Geometry: see drawing. Coordinates: mm, zero at the bounding-box minimum. A direction names the side the tool comes from. Give positions to 0.01 mm unless a question says otherwise; leave off trailing zeros. Write each loop counter-clockwise with the first axis right and the second up, starting at its lowest first coordinate (ties: lowest second). Pieces come first, ordered by that corner, then holes. Notation, with made-up numbers: (49, 52) - (76, 52) arc R33 cw to (76, 85) - close; hole circle Ø3 at (58, 43.5). An arc over 180 degrees is marked (long way). Return JSON: item names as keys, results as strings.
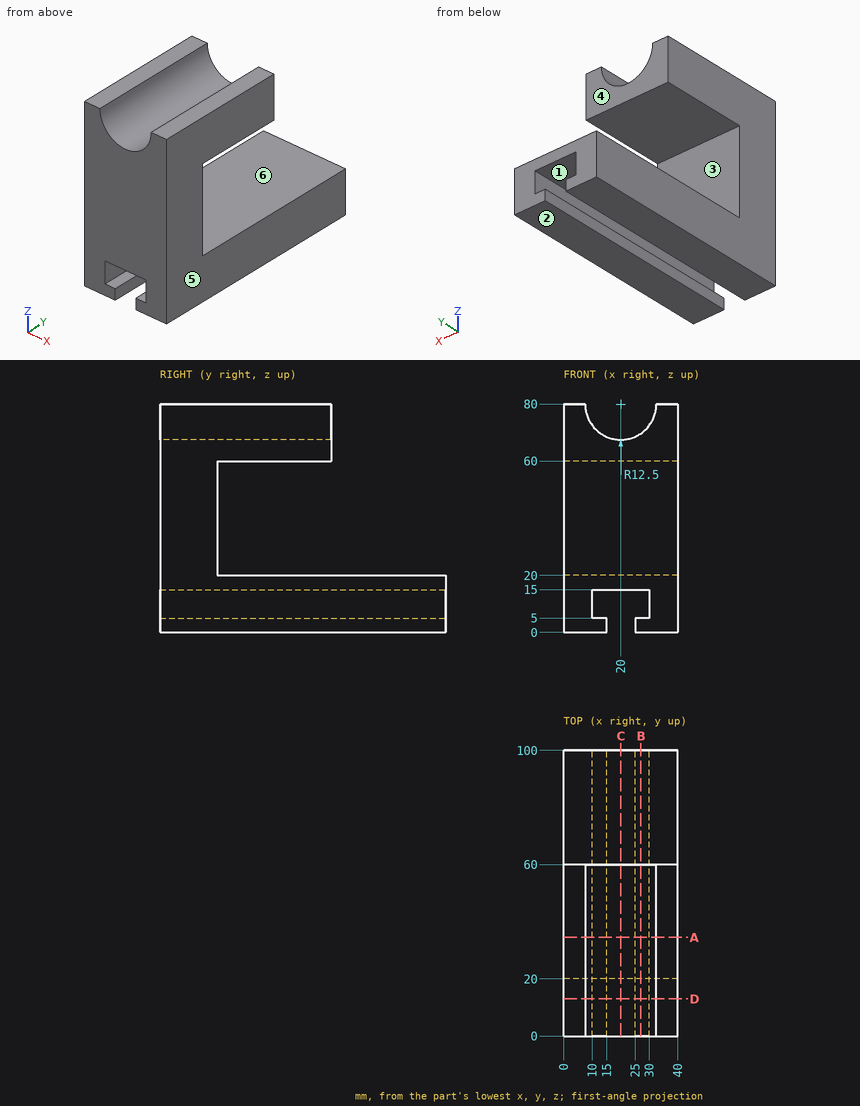
Q1. Section query D-D, the plane y = 13. Return the cut outline in (x, z).
Answer key:
{"outline": "(0, 0) - (15, 0) - (15, 5) - (10, 5) - (10, 15) - (30, 15) - (30, 5) - (25, 5) - (25, 0) - (40, 0) - (40, 80) - (32.5, 80) arc R12.5 cw to (7.5, 80) - (0, 80) - close"}
Q2. Section query B-B, the plane x = 27. Return the cut outline in (y, z).
Answer key:
{"outline": "(0, 0) - (100, 0) - (100, 5) - (0, 5) - close; (0, 15) - (100, 15) - (100, 20) - (20, 20) - (20, 60) - (60, 60) - (60, 69.64) - (0, 69.64) - close"}
Q3. Section query A-A, the plane y = 34.5. Return the cut outline in (x, z), plus the area to 3 significant figures.
Answer key:
{"outline": "(0, 0) - (15, 0) - (15, 5) - (10, 5) - (10, 15) - (30, 15) - (30, 5) - (25, 5) - (25, 0) - (40, 0) - (40, 20) - (0, 20) - close; (0, 60) - (40, 60) - (40, 80) - (32.5, 80) arc R12.5 cw to (7.5, 80) - (0, 80) - close", "area": "1,100 mm^2"}
Q4. Mould query, pull axis Z, two halves, no side actions, for the marked faces 1, 2, 3 and 4. Classes: pulls with the +Z half, pulls with the -Z half, needs draft (parallel to the pull), parting line crosses it, or undercut.
Answer key:
{"face 1": "undercut", "face 2": "pulls with the -Z half", "face 3": "undercut", "face 4": "needs draft"}
Q5. Set-up query: the marked faces 5 and 6. Return all of +Z, -Z, +X, -X, +Y, -Y with unobstructed straight access to the full face (end or side cutting, diameter ignored); none if empty.
Answer key:
{"face 5": "+Z, -Z, +X, +Y, -Y", "face 6": "+X, -X, +Y"}
Q6. Material intervals for probe 1 along Z at (x, y) = (4, 36); probe 2 along Z at (x, y) = (10.5, 57.5); probe 3 along Z at (x, y) = (14.5, 32), sorted ascending. Write a range as [from, to].
Answer key:
{"probe 1": "z = [0, 20], [60, 80]", "probe 2": "z = [0, 5], [15, 20], [60, 71.88]", "probe 3": "z = [0, 5], [15, 20], [60, 68.78]"}
Q7. Pin query (flat end, axial travel): P1, Ø10, axis at x = 13.5, y = 15, coming from the +Z side; P2, Ø10, axis at x = 13, z = 70, coming from the +Y side; P3, Ø2, axis at x = 9, z = 31.5, coming from the +Y side. Return the tip coordinate at first contact, or that it passes through.
Answer key:
{"P1": "stops at z = 75.1", "P2": "stops at y = 60", "P3": "stops at y = 20"}
Q8. Section query C-C, the plane x = 20. Return the cut outline in (y, z).
Answer key:
{"outline": "(0, 15) - (100, 15) - (100, 20) - (20, 20) - (20, 60) - (60, 60) - (60, 67.5) - (0, 67.5) - close"}
